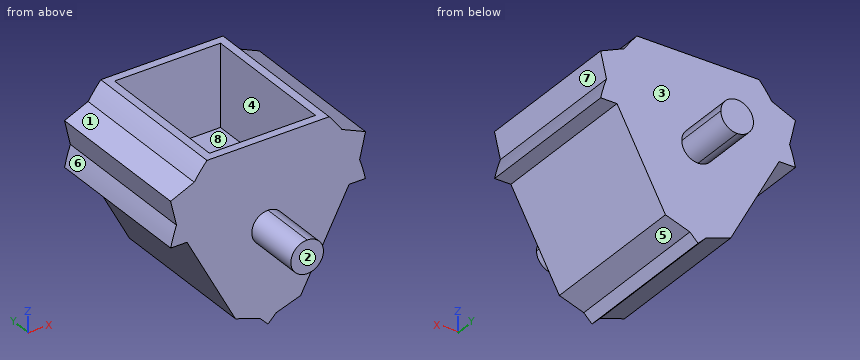
```python
from build123d import *

# Parameters (mm, degrees)
BOSS_EXTRUDE1_DEPTH = 19
BOSS_EXTRUDE2_DEPTH = 7
BOSS_EXTRUDE3_DEPTH = 7
BOSS_EXTRUDE4_DEPTH = 19
CUT_EXTRUDE1_DEPTH  = 19
CUT_EXTRUDE2_DEPTH  = 19
BOSS_EXTRUDE5_DEPTH = 19
BOSS_EXTRUDE6_DEPTH = 19
BOSS_EXTRUDE7_DEPTH = 19
BOSS_EXTRUDE8_DEPTH = 19
BOSS_EXTRUDE9_DEPTH = 19
SKETCH14_W          = 13
SKETCH14_H          = 17
CUT_EXTRUDE3_DEPTH  = 10


with BuildPart() as part:
    # Sketch1 → Boss-Extrude1 (new body)
    with BuildSketch(Plane(origin=(0, 0, 0), x_dir=(1, 0, 0), z_dir=(0, 1, 0))):
        Polygon((4, 0), (7.5, -20), (-7.5, -20), (-4, 0), align=None)
        Polygon((-7.5, -20), (-5.948577014, -11.134725796), (-10.948577014, -11.134725796), (-9.949358248, -13.703422483), (-9.224288507, -15.567362898), (-8.499218766, -17.431303313), align=None)
        Polygon((-9.224288507, -15.567362898), (-9.949358248, -13.703422483), (-11.088228922, -16.292432639), align=None)
        Polygon((-11.088228922, -16.292432639), (-8.499218766, -17.431303313), (-9.224288507, -15.567362898), align=None)
        Polygon((5.948577014, -11.134725796), (7.5, -20), (8.499218766, -17.431303313), (9.224288507, -15.567362898), (9.949358248, -13.703422483), (10.948577014, -11.134725796), align=None)
        Polygon((9.949358248, -13.703422483), (9.224288507, -15.567362898), (11.088228922, -16.292432639), align=None)
        Polygon((9.224288507, -15.567362898), (8.499218766, -17.431303313), (11.088228922, -16.292432639), align=None)
        Polygon((0, 1), (-2, 0), (2, 0), align=None)
    extrude(amount=BOSS_EXTRUDE1_DEPTH)

    # Sketch2 → Boss-Extrude2 (add)
    with BuildSketch(Plane(origin=(0, 19, 0), x_dir=(1, 0, 0), z_dir=(0, 1, 0))):
        with BuildLine():
            ThreePointArc((2, -9.5), (1.414213562, -8.085786438), (0, -7.5))
            Line((0, -7.5), (0, -11.5))
            ThreePointArc((0, -11.5), (1.414213562, -10.914213562), (2, -9.5))
        make_face()
        with BuildLine():
            Line((0, -11.5), (0, -7.5))
            ThreePointArc((0, -7.5), (-2, -9.5), (0, -11.5))
        make_face()
    extrude(amount=BOSS_EXTRUDE2_DEPTH)

    # Sketch3 → Boss-Extrude3 (add)
    with BuildSketch(Plane.XZ):
        with BuildLine():
            ThreePointArc((0, 11.5), (-2, 9.5), (0, 7.5))
            Line((0, 7.5), (0, 11.5))
        make_face()
        with BuildLine():
            Line((0, 11.5), (0, 7.5))
            ThreePointArc((0, 7.5), (1.414213562, 8.085786438), (2, 9.5))
            ThreePointArc((2, 9.5), (1.414213562, 10.914213562), (0, 11.5))
        make_face()
    extrude(amount=BOSS_EXTRUDE3_DEPTH)

    # Sketch4 → Boss-Extrude4 (add)
    with BuildSketch(Plane.XZ):
        Polygon((9.948577014, 11.134725796), (4, 0), (5.948577014, 11.134725796), align=None)
        Polygon((-5.948577014, 11.134725796), (-9.948577014, 11.134725796), (-4, 0), align=None)
    extrude(amount=-BOSS_EXTRUDE4_DEPTH)

    # Sketch5 → Cut-Extrude1 (cut)
    with BuildSketch(Plane.XZ):
        Polygon((9.949358248, 13.703422483), (8.499218766, 17.431303313), (11.088228922, 16.292432639), align=None)
    extrude(amount=-CUT_EXTRUDE1_DEPTH, mode=Mode.SUBTRACT)

    # Sketch6 → Cut-Extrude2 (cut)
    with BuildSketch(Plane.XZ):
        Polygon((-9.949358248, 13.703422483), (-8.499218766, 17.431303313), (-11.088228922, 16.292432639), align=None)
    extrude(amount=-CUT_EXTRUDE2_DEPTH, mode=Mode.SUBTRACT)

    # Sketch7 → Boss-Extrude5 (add)
    with BuildSketch(Plane.XZ):
        Polygon((10.948577014, 11.134725796), (11.948577014, 11.134725796), (7.5, 20), align=None)
        Polygon((-11.948577014, 11.134725796), (-7.5, 20), (-10.948577014, 11.134725796), align=None)
    extrude(amount=-BOSS_EXTRUDE5_DEPTH)

    # Sketch8 → Boss-Extrude6 (add)
    with BuildSketch(Plane.XZ):
        Polygon((2, 0), (0, -2), (-2, 0), (0, -1), align=None)
    extrude(amount=-BOSS_EXTRUDE6_DEPTH)

    # Sketch9 → Boss-Extrude7 (add)
    with BuildSketch(Plane.XZ):
        Polygon((-1, -1), (-4, 0), (-2, 0), align=None)
        Polygon((1, -1), (4, 0), (2, 0), align=None)
    extrude(amount=-BOSS_EXTRUDE7_DEPTH)

    # Sketch10 → Boss-Extrude8 (add)
    with BuildSketch(Plane.XZ):
        Polygon((11.069784798, 12.886012542), (11.958747137, 16.688609807), (8.378792216, 18.248713254), align=None)
        Polygon((-8.378792216, 18.248713254), (-11.069784798, 12.886012542), (-11.958747137, 16.688609807), align=None)
    extrude(amount=-BOSS_EXTRUDE8_DEPTH)

    # Sketch13 → Boss-Extrude9 (add)
    with BuildSketch(Plane.XZ):
        with BuildLine():
            Line((11.069784798, 12.886012542), (11.948577014, 11.134725796))
            ThreePointArc((11.948577014, 11.134725796), (11.633851427, 12.384363188), (11.239303029, 13.61113838))
            Line((11.239303029, 13.61113838), (11.069784798, 12.886012542))
        make_face()
        with BuildLine():
            Line((7.5, 20), (8.378792216, 18.248713254))
            Line((8.378792216, 18.248713254), (9.061461884, 17.951213613))
            ThreePointArc((9.061461884, 17.951213613), (8.313750457, 19.000772297), (7.5, 20))
        make_face()
        with BuildLine():
            Line((-9.061461884, 17.951213613), (-8.378792216, 18.248713254))
            Line((-8.378792216, 18.248713254), (-7.5, 20))
            ThreePointArc((-7.5, 20), (-8.313750457, 19.000772297), (-9.061461884, 17.951213613))
        make_face()
        with BuildLine():
            ThreePointArc((-11.239303029, 13.61113838), (-11.633851427, 12.384363188), (-11.948577014, 11.134725796))
            Line((-11.948577014, 11.134725796), (-11.069784798, 12.886012542))
            Line((-11.069784798, 12.886012542), (-11.239303029, 13.61113838))
        make_face()
    extrude(amount=-BOSS_EXTRUDE9_DEPTH)

    # Sketch14 → Cut-Extrude3 (cut)
    with BuildSketch(Plane.XY.offset(20)):
        with Locations((0, 9.5)):
            Rectangle(SKETCH14_W, SKETCH14_H)
    extrude(amount=-CUT_EXTRUDE3_DEPTH, mode=Mode.SUBTRACT)


solid = part.part
```
Input: part model. Units: mm. Frame: model coordinates. Face numbers are marked on the shaded views. A direction names the side the tool comes from. Give positions to 0.01 mm unless a question says otherwise; leave off trailing zeros. Order: outer loops, then holes, each group sorted by start corner. A loop starts at its lowest first (then second) coordinate and runs counter-clockwise, first axis right, second up. Notation, with made-up numbers: (-10.5, 5.25) - (2.5, 5.25) arc R10 ccw to (2.5, 19.25) - close; hole circle Ø6 at (2.25, 31.5). An arc over 180 degrees is marked (long way). Use a Markdown table: item, result.
(1) Line query: line 1 (Y direction, x = 1.5, z = 11.75); line 2 (Y direction, x = 1.5, z = 10.25); line 3 (Y direction, x = 2, z = 0). Output: solid intervals per line, ascending. Write a range as from..to.
Computed values:
| item | result |
|---|---|
| line 1 | y = 0..1, 18..19 |
| line 2 | y = -7..1, 18..26 |
| line 3 | y = 0..19 |
(2) Section query C-C (z = 8). Output: boundary loops of the cut face in (x, y).
Computed values:
| item | result |
|---|---|
| outline | (-8.27, 0) - (-1.32, 0) - (-1.32, -7) - (1.32, -7) - (1.32, 0) - (8.27, 0) - (8.27, 19) - (1.32, 19) - (1.32, 26) - (-1.32, 26) - (-1.32, 19) - (-8.27, 19) - close |
(3) Access query for the marked faces 5, 6, 7 and 8. Directions: +Z, -Z, +X, -X, +Y, -Y. A direction counts if a zero-diameter tool reaches every point of the face in a straight line with its end or side. Return the directions, or none.
Computed values:
| item | result |
|---|---|
| face 5 | -Z, +X, +Y, -Y |
| face 6 | -X, +Y, -Y |
| face 7 | +X, +Y, -Y |
| face 8 | +Z |
(4) Draft query along Y for the marked faces 1, 2, 3 and 4. Return one class per face: released by +Y, released by -Y, zero draft, split by the parting line, or undercut.
Computed values:
| item | result |
|---|---|
| face 1 | zero draft |
| face 2 | released by -Y |
| face 3 | released by +Y |
| face 4 | undercut |
(5) Pin query (flat end, axial travel): pin 1 (5 mm diameter, centred on x = 2, y = 9, fed in from -Z); pin 2 (1 mm diameter, centred on x = -11, y = 12, fed in from -Z); pin 3 (6.5 mm diameter, centred on x = 1.5, y = 11.5, fed in from +Z); pin 4 (10 mm diameter, centred on x = -3.5, z = 2.5, fed in from -Y). Return the tip coordinate at first contact, or that it passes through.
Computed values:
| item | result |
|---|---|
| pin 1 | stops at z = -2 |
| pin 2 | stops at z = 11.13 |
| pin 3 | stops at z = 10 |
| pin 4 | stops at y = 0 |
(6) Section query D-D (y = -2.5). Output: boundary loops of the cut face in (x, z).
Computed values:
| item | result |
|---|---|
| outline | circle Ø4 at (0, 9.5) |
(7) Section query B-B (x = -3.25). Output: boundary loops of the cut face in (y, z), then the cut area to 3 significant figures.
Computed values:
| item | result |
|---|---|
| outline | (0, -0.25) - (19, -0.25) - (19, 20) - (18, 20) - (18, 10) - (1, 10) - (1, 20) - (0, 20) - close |
| area | 215 mm2 |
(8) Section query A-A (y = 15.5). Output: boundary loops of the cut face in (x, z), then the cut area to 3 significant figures.
Computed values:
| item | result |
|---|---|
| outline | (-11.96, 16.69) - (-11.24, 13.61) arc R20 ccw to (-11.95, 11.13) - (-9.95, 11.13) - (-4, 0) - (-1, -1) - (0, -2) - (1, -1) - (4, 0) - (9.95, 11.13) - (11.95, 11.13) arc R20 ccw to (11.24, 13.61) - (11.96, 16.69) - (9.06, 17.95) arc R20 ccw to (7.5, 20) - (6.5, 20) - (6.5, 10) - (-6.5, 10) - (-6.5, 20) - (-7.5, 20) arc R20 ccw to (-9.06, 17.95) - close |
| area | 221 mm2 |
